```python
from build123d import *

# Parameters (mm, degrees)
SKETCH1_R           = 6.35
SKETCH1_R_2         = 6.6675
BOSS_EXTRUDE1_DEPTH = 9.525
SKETCH2_W           = 21.59
SKETCH2_H           = 20.921938848
CUT_EXTRUDE1_DEPTH  = 3.302
CUT_EXTRUDE2_DEPTH  = 4.953


with BuildPart() as part:
    # Sketch1 → Boss-Extrude1 (new, symmetric)
    with BuildSketch(Plane(origin=(0, 0, 0), x_dir=(1, 0, 0), z_dir=(0, 1, 0))):
        with BuildLine():
            Line((-0.79375, 9.491869465), (37.041666667, 12.655825953))
            ThreePointArc((37.041666667, 12.655825953), (50.8, 0), (37.041666667, -12.655825953))
            Line((37.041666667, -12.655825953), (-0.79375, -9.491869465))
            ThreePointArc((-0.79375, -9.491869465), (-9.525, 0), (-0.79375, 9.491869465))
        make_face()
        Circle(SKETCH1_R, mode=Mode.SUBTRACT)
        with Locations((38.1, 0)):
            Circle(SKETCH1_R_2, mode=Mode.SUBTRACT)
    extrude(amount=BOSS_EXTRUDE1_DEPTH, both=True)

    # Sketch2 → Cut-Extrude1 (cut, symmetric)
    with BuildSketch(Plane(origin=(0, 0, 0), x_dir=(1, 0, 0), z_dir=(0, 1, 0))):
        Rectangle(SKETCH2_W, SKETCH2_H)
    extrude(amount=CUT_EXTRUDE1_DEPTH, both=True, mode=Mode.SUBTRACT)

    # Sketch3 → Cut-Extrude2 (cut, symmetric)
    with BuildSketch(Plane(origin=(0, 0, 0), x_dir=(1, 0, 0), z_dir=(0, 1, 0))):
        with BuildLine():
            Line((37.041666667, 12.655825953), (16.4, 10.929683071))
            Line((16.4, 10.929683071), (16.4, -10.929683071))
            Line((16.4, -10.929683071), (37.041666667, -12.655825953))
            ThreePointArc((37.041666667, -12.655825953), (50.8, 0), (37.041666667, 12.655825953))
        make_face()
    extrude(amount=CUT_EXTRUDE2_DEPTH, both=True, mode=Mode.SUBTRACT)


solid = part.part
```
For this review, take the finished solid that the model builds, in its own axes (mm). A direction names the side the tool comes from. Round coordinates to 2 decimals unless told otherwise and drop trailing zeros. Write each loop counter-clockwise with the first axis right and the second up, starting at its lowest first coordinate (ties: lowest second). Pieces come first, ordered by that corner, then holes. Notation, with made-up numbers: (43.5, 75.5) -> (100.5, 75.5) arc R21 cw to (100.5, 93.5) -> close; hole circle Ø5 at (-6.75, 46). An arc over 180 degrees is marked (long way). Use one line per item in the form item = value.
Q1. Consider section B-B (y = 8). State how many separate pieces and enclosed holes the cut face has, then the cut area to 3 significant figures.
Resolved:
separate_pieces = 1
enclosed_holes = 2
area = 979 mm²
Q2. The part is to be moulded in two halves that separate along Z. For faces 1 (the flat face through (14.185, 0.133, 10.744)), 2 (the flat face through (30, 4.953, 0)), 3 (the cylindrical face through (31.44, 7.21, -0.29)), 4 (the cylindrical face through (50.797, -7.207, -0.294)), say which applies: released by +Z, released by -Z, zero draft, split by the parting line, or undercut.
Resolved:
face_1 = released by +Z
face_2 = zero draft
face_3 = undercut
face_4 = split by the parting line
Q3. Machinability: for faces 5 (the flat face through (10.795, 0, 0)), 6 (the flat face through (16.4, 0, 0)), 7 (the cylindrical face through (-1.38, -6.46, 6.2)), which of the approach directions +Z, -Z, +X, -X, +Y, -Y give a long, thin tool a straight path to every point of the face, cutting with its end or side? Answer none if there is none.
Resolved:
face_5 = +Z, -Z, -X
face_6 = +Z, -Z, +X
face_7 = +Y, -Y
Q4. Clearance check with flat-ended pins moving along their axes: pin 1 Ø6 at (x, y) = (6.5, 5.5) entering from +Z; pin 2 Ø8 at (x, y) = (27, 2) entering from -Z; pin 3 Ø5 at (y, z) = (-0.5, -6) entering from -X (3 decimals). State where each tip first meets the part, or that it passes through.
Resolved:
pin_1 = 10.35
pin_2 = -12.04
pin_3 = 10.795
Q5. To check wall thickness, follow probe 1 along Y at (x, z) = (20, 7.75) (3 decimals); probe 2 along X at (y, z) = (5.5, -2.75); probe 3 along Y at (x, z) = (5.5, -9) (3 decimals). State the ranges of each line that lie inside material, in increasing order. Write a range as from..to.
Resolved:
probe_1 = -9.525..-4.953, 4.953..9.525
probe_2 = -9.12..-5.72, 5.72..32.03, 44.17..50.5
probe_3 = -9.525..-3.302, 3.302..9.525
Q6. Consider section A-A (x = 38.1). State the section outline as (y, z) points (1 decimal).
Resolved:
outline = (-9.5, -12.7) -> (-5, -12.7) -> (-5, -6.7) -> (-9.5, -6.7) -> close; (-9.5, 6.7) -> (-5, 6.7) -> (-5, 12.7) -> (-9.5, 12.7) -> close; (5, -12.7) -> (9.5, -12.7) -> (9.5, -6.7) -> (5, -6.7) -> close; (5, 6.7) -> (9.5, 6.7) -> (9.5, 12.7) -> (5, 12.7) -> close
Q7. Consider section D-D (y = -4). State the section outline as (x, z) points (3 decimals), then the cut area to 3 significant figures.
Resolved:
outline = (-0.794, -9.492) -> (16.4, -10.93) -> (16.4, 10.93) -> (-0.794, 9.492) arc R9.525 ccw to start; hole circle Ø12.7 at (0, 0)
area = 352 mm²
